Design review of the part built by this model. Coordinates are the model's own, in mm. A direction names the side the tool comes from. Give positions to 0.01 mm unless a question says otherwise; leave off trailing zeros. Order: outer loops, then holes, each group sorted by start corner. A loop starts at its lowest first (then second) coordinate and runs counter-clockwise, first axis right, second up. Notation, with made-up numbers: (-2, -11.75) - (31, -11.75) arc R30 ccw to (31, 15.25) - close; hole circle Ø6 at (-27.5, 5). An arc over 180 degrees is marked (long way). Write each question's results on one line, items separated by ' | '. Start each with the question number.
Autodesk Inventor part; units mm, degrees
ref_plane "YZ Plane" through (0, 0, 0) normal (1, 0, 0) x (0, 1, 0)
ref_plane "XZ Plane" through (0, 0, 0) normal (0, 1, 0) x (-1, 0, 0)
ref_plane "XY Plane" through (0, 0, 0) normal (0, 0, 1) x (1, 0, 0)
sketch "Sketch1" plane through (0, 0, 0) normal (0, 0, 1) x (1, 0, 0)
  line L0 (17, 4.5) -> (17, -4.5)
  line L1 (-17, -4.5) -> (-17, 4.5)
  arc A0 (-8.3666, -4.5) -> (8.3666, -4.5) centre (0, 0) ccw
  arc A1 (8.3666, 4.5) -> (-8.3666, 4.5) centre (0, 0) ccw
  line L2 (-17, 4.5) -> (-8.3666, 4.5)
  line L3 (8.3666, 4.5) -> (17, 4.5)
  line L4 (17, -4.5) -> (8.3666, -4.5)
  line L5 (-8.3666, -4.5) -> (-17, -4.5)
  line L6 (-17, 4.5) -> (17, -4.5) construction
  line L7 (-17, -4.5) -> (17, 4.5) construction
  point P0 (0, 0)
  point P1 (0, 0)
  dimension "d0" = 9
  dimension "d1" = 34
  dimension "d2" = 9.5
  dimension "d3" = 9
  dimension "d4" = 9.5
  dimension "d12" = 4.5
extrude "Extrusion1" add sketch "Sketch1" along normal blind 7
sketch "Sketch2" plane through (17, -4.5, 0) normal (1, 0, 0) x (0, 0, -1)
  arc A0 (-11.5, 9) -> (-11.5, 0) centre (-11.5, 4.5) ccw
  circle A1 centre (-11.5, 4.5) radius 2.25
  line L0 (-7, 9) -> (-11.5, 9)
  line L1 (-11.5, 0) -> (-7, 0)
  line L2 (-7, 0) -> (-7, 9)
  point P0 (0, 4.5)
  point P1 (-7, 0)
  dimension "d7" = 9
  dimension "d8" = 4.5
  dimension "d9" = 9
extrude "Extrusion2" add sketch "Sketch2" against normal blind 4.3
extrude "Extrusion3" add sketch "Sketch2" along normal blind 4.3 from surface at -34
sketch "Sketch3" plane through (-17, -4.5, 0) normal (0, -1, 0) x (1, 0, 0)
  line L0 (0, 6) -> (0, 0)
  line L1 (0, 0) -> (5, 0)
  line L2 (5, 0) -> (0, 6)
  line L3 (29, 0) -> (34, 0)
  line L4 (34, 0) -> (34, 6)
  line L5 (34, 6) -> (29, 0)
  point P0 (17, 0)
  dimension "d15" = 6
  dimension "d16" = 5
  dimension "d17" = 6
  dimension "d18" = 5
extrude "Extrusion4" cut sketch "Sketch3" against normal up to next
sketch "Sketch4" plane through (0, 0, 0) normal (0, 0, -1) x (-1, 0, 0)
  circle A0 centre (0, 0) radius 7.5
  dimension "d21" = 15
extrude "Extrusion5" add sketch "Sketch4" along normal blind 2.5
sketch "Sketch5" plane through (0, 0, 7) normal (0, 0, 1) x (1, 0, 0)
  circle A0 centre (0, 0) radius 7.5
  dimension "d24" = 15
extrude "Extrusion6" cut sketch "Sketch5" against normal blind 4
sketch "Sketch6" plane through (0, 0, -2.5) normal (0, 0, -1) x (-1, 0, 0)
  circle A0 centre (0, 0) radius 5.5
  dimension "d27" = 11
extrude "Extrusion7" cut sketch "Sketch6" against normal blind 4
sketch "Sketch7" plane through (0, 0, 1.5) normal (0, 0, -1) x (-1, 0, 0)
  circle A0 centre (0, 0) radius 5
  dimension "d30" = 10
extrude "Extrusion8" cut sketch "Sketch7" against normal up to next
sketch "Sketch9" plane through (0, 0, 0) normal (1, 0, 0) x (0, 1, 0)
  arc A0 (31.2893, 14.3034) -> (30.2107, 19.6966) centre (30.75, 17) ccw
  line L0 (-9.5504, 0) -> (57.3026, 0)
  line L1 (0, -37.6235) -> (0, 29.8791)
  circle A1 centre (30.75, 17) radius 1.25
  arc A2 (25.2107, 18.6966) -> (23.9154, 18.0486) centre (25.75, 16) ccw
  circle A3 centre (25.75, 16) radius 1.25
  line L2 (9.5, 7) -> (9.5, 0)
  line L3 (9.5, 0) -> (12.3425, 0)
  line L4 (25.2107, 18.6966) -> (30.2107, 19.6966)
  line L5 (26.2893, 13.3034) -> (31.2893, 14.3034)
  arc A4 (23.9154, 18.0486) -> (9.5, 7) centre (47.7522, -27.9802) ccw
  arc A5 (26.2893, 13.3034) -> (14.061, 0.9769) centre (44.8843, -17.3723) ccw
  arc A6 (12.3425, 0) -> (14.061, 0.9769) centre (12.3425, 2) ccw
  line L6 (8.5, 7) -> (9.5, 7)
  line L7 (9.5, 7) -> (9.5, 0)
  line L8 (9.5, 0) -> (8.5, 0)
  line L9 (8.5, 0) -> (8.5, 7)
  point P0 (0, 0)
  point P1 (13.5, 0)
  dimension "d53" = 5.5
  dimension "d54" = 17
  dimension "d55" = 30.75
  dimension "d56" = 2.5
  dimension "d57" = 16
  dimension "d58" = 25.75
  dimension "d59" = 4
  dimension "d60" = 7
  dimension "d61" = 9.5
  dimension "d62" = 0
  dimension "d63" = 51.8348
  dimension "d64" = 35.8716
  dimension "d65" = 2
  dimension "d88" = 7
  dimension "d89" = 1
  dimension "d90" = 0
  dimension "d91" = 0
extrude "Extrusion9" add sketch "Sketch9" along normal mid plane 4 contours L5 A5 A6 L0 L2 A4 A2 L4 A0
sketch "Sketch10" plane through (0, 0, 0) normal (1, 0, 0) x (0, 1, 0)
  arc A0 (25.2107, 18.6966) -> (26.2893, 13.3034) centre (25.75, 16) ccw
  circle A1 centre (25.75, 16) radius 1.25
  arc A2 (31.2893, 14.3034) -> (30.2107, 19.6966) centre (30.75, 17) ccw
  circle A3 centre (25.75, 16) radius 1.25
  circle A4 centre (30.75, 17) radius 1.25
  circle A5 centre (30.75, 17) radius 1.25
  line L0 (25.2107, 18.6966) -> (30.2107, 19.6966)
  line L1 (26.2893, 13.3034) -> (31.2893, 14.3034)
  point P0 (0, 0)
  dimension "d68" = 5.5
  dimension "d69" = 2.5
extrude "Extrusion10" add sketch "Sketch10" along normal blind 3.5
sketch "Sketch11" plane through (0, 0, 0) normal (1, 0, 0) x (0, 1, 0)
  line L0 (-4.2102, 0) -> (25.2612, 0)
  line L1 (0, -2.5102) -> (0, 15.0612)
  line L2 (19.9196, 12.551) -> (11.6686, 4.3)
  line L3 (11.6686, 4.3) -> (0, 4.3)
  line L4 (21.051, 11.4196) -> (12.3314, 2.7)
  line L5 (12.3314, 2.7) -> (0, 2.7)
  line L6 (21.051, 11.4196) -> (19.9196, 12.551)
  line L7 (0, 4.3) -> (0, 2.7)
  point P0 (0, 0)
extrude "Extrusion11" add sketch "Sketch11" along normal mid plane 12
extrude "Extrusion12" cut sketch "Sketch5" against normal blind 4
extrude "Extrusion13" cut sketch "Sketch7" against normal through all
sketch "Sketch12" plane through (0, 0, 0) normal (0, 0, 1) x (1, 0, 0)
  line L0 (6, 7.3655) -> (6, 12.3314)
  line L1 (2, 21.051) -> (6, 21.051)
  arc A0 (6, 7.3655) -> (2, 21.051) centre (-49.0316, -1.2919) ccw
  line L2 (0, 0) -> (0, 16.5543) construction
  arc A1 (-2, 21.051) -> (-6, 7.3655) centre (49.0316, -1.2919) ccw
  line L3 (2, 14.061) -> (2, 14.061) construction
  line L4 (2, 21.051) -> (6, 21.051)
  line L5 (6, 7.3655) -> (6, 21.051)
  line L6 (-6, 7.3655) -> (-6, 21.051)
  line L7 (-2, 21.051) -> (-6, 21.051)
  point P0 (2, 26.2893)
extrude "Extrusion14" cut sketch "Sketch12" along normal up to next
sketch "Sketch13" plane through (0, 0, 0) normal (1, 0, 0) x (0, 1, 0)
  line L0 (8.5, 7) -> (9.5, 7)
  line L1 (9.5, 7) -> (9.5, 0)
  line L2 (9.5, 0) -> (8.5, 0)
  line L3 (8.5, 0) -> (8.5, 7)
  line L4 (0, -6.95) -> (0, 24.2)
  line L5 (-18.1, 0) -> (42.1, 0)
  point P0 (0, 0)
  dimension "d92" = 7
  dimension "d93" = 1
  dimension "d94" = 9.5
  dimension "d95" = 0
extrude "Extrusion15" add sketch "Sketch13" along normal mid plane 4
properties part number "RCT-P006_steering_knuckle"
Q1. For line 1 (X direction, y = 1.5, z = 13.5); line 2 (Y direction, x = 0, z = 2.1); line 3 (Y direction, x = 14.25, z = 11.5), list the stretches that pass through material, from the lowest coordinate up. Write a range as [from, to].
Q2. Add section B-B (y = 0). Give the number of separate pieces and of enclosed holes in the cut face, plus the area to 3 significant figures.
Q3. Draft analysis for pull direction X (two halves, no side actions). For faces 1 (the flat face through (-1.6, -4.9, 1.5)), 2 (the flat face through (0.712, 28.754, 13.796)), 3 (the cylindrical face through (0.1, -9.5, 3.5)), state which applies: pulls with the +X half, pulls with the -X half, needs draft (parallel to the pull), parting line crosses it, or undercut.
Q4. Add section C-C (z = 6.5). Give the boundary of the cut face in (x, y), plus the area to 3 significant figures.
Q5. Add section D-D (x = -14.5). Give the boundary of the cut face in (y, z), plus the area to 3 significant figures.
Q6. Add section A-A (x = 0). Give the boundary of the cut face in (y, z), plus the area to 3 significant figures.
Q7. Machinability: for faces 4 (the flat face through (-3.25, 14.94, 7.57)), 5 (the flat face through (3.14, 15.78, 6.15)), 6 (the flat face through (-3.18, 15.78, 6.15)), 7 (the cylindrical face through (6.37, 7.05, 3.45)), which of the approach directions +Z, -Z, +X, -X, +Y, -Y give a long, thin tool a straight path to every point of the face, cutting with its end or side? Answer none if there is none.
Q8. Insertion check: pin 1 Ø8 at (x, z) = (-6, 9.5) entering from -Y; pin 2 Ø1.9 at (y, z) = (28, 15.5) entering from +X; pin 3 Ø4 at (y, z) = (17.5, 6) entering from +X. Each pin has a flat end and moves straight along its axis. Give the tip position at first contact, or say it passes through.
Verdict:
1) line 1: x = [-17, -12.7], [12.7, 17] | line 2: y = [-9.5, -5], [5, 14.76] | line 3: y = [-4.5, -2.25], [2.25, 4.5]
2) separate pieces: 4 | enclosed holes: 0 | area: 165 mm2
3) face 1: undercut | face 2: needs draft | face 3: parting line crosses it
4) outline: (-17, -4.5) - (-8.37, -4.5) arc R9.5 ccw to (8.37, -4.5) - (17, -4.5) - (17, 4.5) - (8.37, 4.5) arc R9.5 ccw to (2, 9.29) - (2, 13.87) - (4.57, 13.87) arc R55.71 ccw to (3.88, 16.13) - (2, 16.13) - (2, 18.11) - (-2, 18.11) - (-2, 16.13) - (-3.88, 16.13) arc R55.71 ccw to (-4.57, 13.87) - (-2, 13.87) - (-2, 9.29) arc R9.5 ccw to (-8.37, 4.5) - (-17, 4.5) - close; hole circle Ø15 at (0, 0) | area: 293 mm2
5) outline: (-4.5, 3) - (4.5, 3) - (4.5, 11.5) arc R4.5 ccw to (-4.5, 11.5) - close; hole circle Ø4.5 at (0, 11.5) | area: 92.4 mm2
6) outline: (-9.5, 0) - (-7.5, 0) - (-7.5, -2.5) - (-5.5, -2.5) - (-5.5, 1.5) - (-5, 1.5) - (-5, 3) - (-7.5, 3) - (-7.5, 7) - (-9.5, 7) - close; (5, 1.5) - (5.5, 1.5) - (5.5, -2.5) - (7.5, -2.5) - (7.5, 0) - (12.34, 0) arc R2 ccw to (14.06, 0.98) arc R35.87 cw to (26.29, 13.3) - (31.29, 14.3) arc R2.75 ccw to (30.21, 19.7) - (25.21, 18.7) arc R2.75 ccw to (23.92, 18.05) arc R51.84 ccw to (9.5, 7) - (7.5, 7) - (7.5, 3) - (5, 3) - close; hole circle Ø2.5 at (25.75, 16); hole circle Ø2.5 at (30.75, 17) | area: 213 mm2
7) face 4: +Z, -X | face 5: -Z, +X, +Y | face 6: -Z, -X, +Y | face 7: +X
8) pin 1: stops at y = -9.05 | pin 2: stops at x = 3.5 | pin 3: stops at x = 4.09
